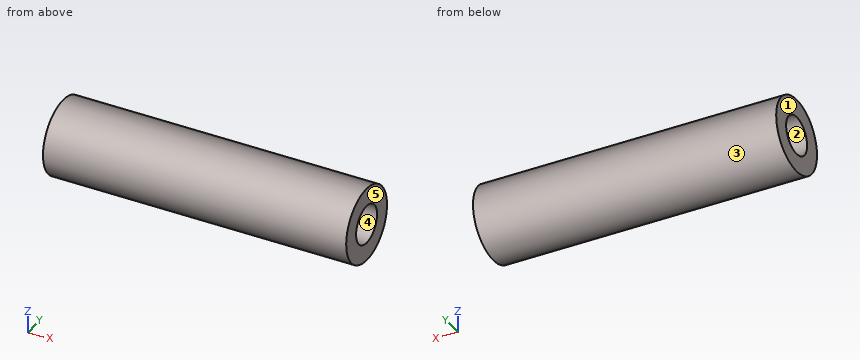
```python
from build123d import *

# Parameters (mm, degrees)
F0_W     = 57
F0_H     = 7
F3_D     = 7.2
F3_DEPTH = 20
F3_TIP   = 2.1630982285
F5_D     = 7.2
F5_DEPTH = 20
F5_TIP   = 2.1630982285


with BuildPart() as f1:
    # F0 (on Front) → F1 (revolve)
    with BuildSketch(Plane.XZ):
        with Locations((0, 3.5)):
            Rectangle(F0_W, F0_H)
    revolve(axis=Axis((-4.6887677163, 0, 0), (1, 0, 0)))

    # F3
    with Locations(Plane.YZ.offset(28.5)):
        with Locations((0, 0)):
            Hole(F3_D / 2, depth=F3_DEPTH)
            with Locations((0, 0, -(F3_DEPTH + F3_TIP / 2))):  # 118° drill point
                Cone(0, F3_D / 2, F3_TIP, mode=Mode.SUBTRACT)

    # F5
    with Locations(Plane(origin=(-28.5, 0, 0), x_dir=(0, -1, 0), z_dir=(-1, 0, 0))):
        with Locations((0, 0)):
            Hole(F5_D / 2, depth=F5_DEPTH)
            with Locations((0, 0, -(F5_DEPTH + F5_TIP / 2))):  # 118° drill point
                Cone(0, F5_D / 2, F5_TIP, mode=Mode.SUBTRACT)


solid = f1.part
```
CAD build for the part. Positions are in the model's coordinates, mm. Face numbers are marked on the shaded views. A direction names the side the tool comes from. Coordinates: 2 decimals unless noted, no trailing zeros. Loops run counter-clockwise (first coordinate to the right, second up) from the corner with the lowest first, then second, coordinate; pieces in that order, holes last. Notation, with made-up numbers: (82.5, 30) - (114.5, 30) arc R20 ccw to (114.5, 43) - close; hole circle Ø4 at (70.25, 23). An arc over 180 degrees is marked (long way). Return JSON: item names as keys, results as strings.
1. Probe L1, parallel to Y at x = 15.25, z = 0; L2, parallel to Z at x = -16, y = 2.5. List the from-to ranges inside material, lowest first. Write a range as from..to.
Result:
{"L1": "y = -7..-3.6, 3.6..7", "L2": "z = -6.54..-2.59, 2.59..6.54"}
2. Band-saw the part on D-D (y = -4.25). Give the cut face in (x, z).
Result:
{"outline": "(-28.5, -5.56) - (28.5, -5.56) - (28.5, 5.56) - (-28.5, 5.56) - close"}
3. Band-saw the part on C-C (x = -5.5). Give the cut face in (y, z).
Result:
{"outline": "circle Ø14 at (0, 0)"}
4. 3-axis set-ups, long thin cutter, end or side, ignore diameter. For the marked faces 4 and 5: which of +Z, -Z, +X, -X, +Y, -Y reach the whole face in a straight line?
Result:
{"face 4": "+X", "face 5": "+Z, -Z, +X, +Y, -Y"}
5. Mould opens along Y. For the marked faces 1, 2 and 3 say: released by +Y, released by -Y, zero draft, split by the parting line, or undercut.
Result:
{"face 1": "zero draft", "face 2": "undercut", "face 3": "split by the parting line"}
6. Drop flat-ended pins along their axis: pin 1 (3 mm diameter, centred on x = -2, z = 4.5, fed in from +Y); pin 2 (4 mm diameter, centred on x = 13.5, y = 4, fed in from -Z). Give the stop position or say it passes through.
Result:
{"pin 1": "stops at y = 6.32", "pin 2": "stops at z = -6.71"}
7. Band-saw the part on A-A (x = 10). Give the cut face in (y, z).
Result:
{"outline": "circle Ø14 at (0, 0); hole circle Ø7.2 at (0, 0)"}
8. Band-saw the part on B-B (z = -4.5). Give the cut face in (x, y), and give its area (3 significant figures).
Result:
{"outline": "(-28.5, -5.36) - (28.5, -5.36) - (28.5, 5.36) - (-28.5, 5.36) - close", "area": "611 mm2"}
